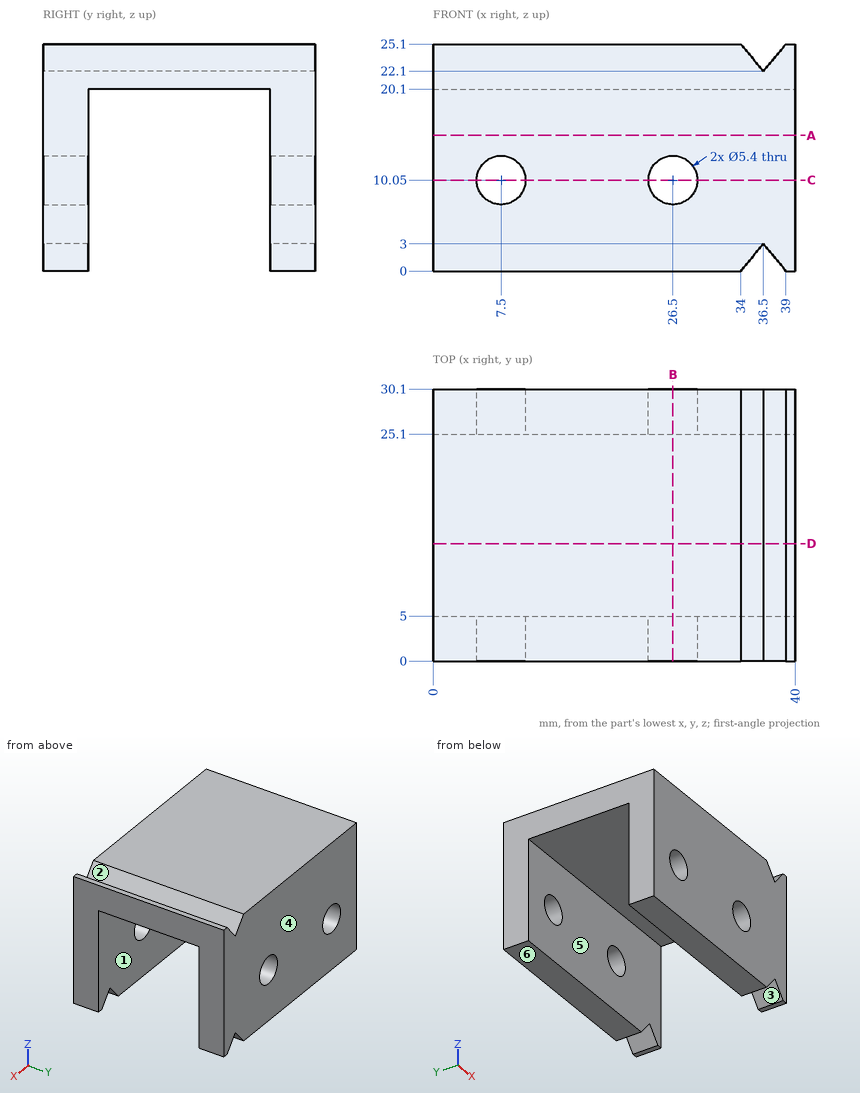
Verification items for this drawing (mm, ordinates from the low corner). A direction names the side the tool comes from. Coordinates: 2 decimals unless noted, no trailing zeros. Order: outer loops, then holes, each group sorted by start corner. A loop starts at its lowest first (then second) coordinate and runs counter-clockwise, first axis right, second up. Notation, with made-up numbers: (19.5, 42) -> (56.5, 42) arc R24 ccw to (56.5, 56) -> close; hole circle Ø7 at (44, 58.5). An arc over 180 degrees is marked (long way). Put each result on its own line as item: value. Start each with the question number.
1. Cross-section at A-A, the plane z = 15. Record the boundary of the cut face in (x, y).
2. Go/stop test with flat-tipped pins: pin 1 Ø5 at (x, z) = (7.5, 10.05) entering from +Y; pin 2 Ø10 at (x, y) = (21.5, 17.5) entering from -Z. Record where each tip stops, or that it passes through.
3. Cross-section at B-B, the plane x = 26.5. Record the boundary of the cut face in (y, z).
4. Cross-section at D-D, the plane y = 13. Record the boundary of the cut face in (x, z), then the cut area to 4 significant figures.
5. Material ranges on L1, parallel to Y at x = 33.5, z = 6.25; L2, parallel to Z at x = 7.5, y = 27.5; L3, parallel to X at y = 3, z = 9.25, recorded low to high. Write a range as [from, to].
6. Access from +Z, -Z, +X, -X, +Y, -Y to the whole of each face (thin tool, end or side, straight path). Record for the marked faces 1, 2 and 3.
7. Cross-section at C-C, the plane z = 10.05. Record the boundary of the cut face in (x, y).
8. Mould release check, pull along Y, two halves, no side actions. Record for the marked faces 4, 5 and 6: released by +Y, released by -Y, zero draft, split by the parting line, or undercut.
Computed:
1. outline: (0, 0) -> (40, 0) -> (40, 5) -> (0, 5) -> close; (0, 25.1) -> (40, 25.1) -> (40, 30.1) -> (0, 30.1) -> close
2. pin 1: through
2. pin 2: z = 20.1
3. outline: (0, 0) -> (5, 0) -> (5, 7.35) -> (0, 7.35) -> close; (0, 12.75) -> (5, 12.75) -> (5, 20.1) -> (25.1, 20.1) -> (25.1, 12.75) -> (30.1, 12.75) -> (30.1, 25.1) -> (0, 25.1) -> close; (25.1, 0) -> (30.1, 0) -> (30.1, 7.35) -> (25.1, 7.35) -> close
4. outline: (0, 20.1) -> (40, 20.1) -> (40, 25.1) -> (39, 25.1) -> (36.5, 22.1) -> (34, 25.1) -> (0, 25.1) -> close
4. area: 192.5 mm2
5. L1: [0, 5], [25.1, 30.1]
5. L2: [0, 7.35], [12.75, 25.1]
5. L3: [0, 4.92], [10.08, 23.92], [29.08, 40]
6. face 1: -Z, +X, -X
6. face 2: +Z, +Y, -Y
6. face 3: -Z, +Y, -Y
7. outline: (0, 0) -> (4.8, 0) -> (4.8, 5) -> (0, 5) -> close; (0, 25.1) -> (4.8, 25.1) -> (4.8, 30.1) -> (0, 30.1) -> close; (10.2, 0) -> (23.8, 0) -> (23.8, 5) -> (10.2, 5) -> close; (10.2, 25.1) -> (23.8, 25.1) -> (23.8, 30.1) -> (10.2, 30.1) -> close; (29.2, 0) -> (40, 0) -> (40, 5) -> (29.2, 5) -> close; (29.2, 25.1) -> (40, 25.1) -> (40, 30.1) -> (29.2, 30.1) -> close
8. face 4: released by +Y
8. face 5: undercut
8. face 6: zero draft
